```python
from build123d import *

# Parameters (mm, degrees)
F1_DEPTH = 17.5
F2_W     = 8
F2_H     = 3
F2_W_2   = 15
F2_H_2   = 1
F3_DEPTH = 50
F5_DEPTH = 2.5


# Not quite as in the source:
# - a pattern or mirror of a feature is missing from the dataset's text; its kind, count and spacing are read off the source's solid


with BuildPart() as f1:
    # F0 (on Front) → F1 (new body, symmetric)
    with BuildSketch(Plane.XZ):
        Polygon((-11.8, 0), (0, 0), (11.8, 0), (11.8, 8), (11, 8), (7.75, 2.5), (0, 2.5), (-7.75, 2.5), (-11, 8), (-11.8, 8), align=None)
    extrude(amount=F1_DEPTH, both=True)

    # F2 (on Right) → F3 (cut, symmetric)
    with BuildSketch(Plane.YZ):
        with Locations((0, 4)):
            Rectangle(F2_W, F2_H)
        with Locations((0, 0.5)):
            Rectangle(F2_W_2, F2_H_2)
    extrude(amount=F3_DEPTH, both=True, mode=Mode.SUBTRACT)

    # F4 (on Top) → F5 (join)
    with BuildSketch(Plane.XY):
        Polygon((26.4065545634, 26.1439538722), (11.8, 17.5), (11.8, 8.5), (27.6797758895, 23.9924642824), align=None)
        Polygon((11.8, -8.5), (11.8, -17.5), (21.2564246661, -23.0961793217), (23.2712739184, -19.6914867497), align=None)
    f5 = extrude(amount=F5_DEPTH)

    # F5_copies: F5 across plane
    add(f5.mirror(Plane(origin=(0, 0, 0), x_dir=(0, 0, -1), z_dir=(-1, 0, 0))))


solid = f1.part
```
Geometry: final body of the model. Coordinates: model frame, mm. A direction names the side the tool comes from. Round coordinates to 2 decimals unless told otherwise and drop trailing zeros. Order: outer loops, then holes, each group sorted by start corner. A loop starts at its lowest first (then second) coordinate and runs counter-clockwise, first axis right, second up. Notation, with made-up numbers: (62, 11) - (121, 11) arc R14 cw to (121, 22) - close; hole circle Ø6 at (57, 42). An arc over 180 degrees is marked (long way). Write item = value, one per line. Start each with the question number.
Q1. Cut plane B-B on z = 6.25. Return the cut outline in (x, y), and give its area (3 significant figures).
Q2. Ray query, line 1 (Z direction, x = -11, y = -2); line 2 (Z direction, x = 1, y = -8); line 3 (X direction, y = -6.5, z = 7.75). Return the intervals inside material, ascending. Write a range as from..to.
Q3. Cut plane D-D on y = -15.5. Return the cut outline in (x, z) (3 decimals).
Q4. Cut plane C-C on x = 17.5. Return the cut outline in (y, z), and give its area (3 significant figures).
Q5. Access query for faces 1 (the flat face through (19, 18, 2.5)), 2 (the flat face through (-16, -17, 2.5)), 3 (the flat face through (0, 0, 1)), 4 (the flat face through (-19.63, 16.14, 1.23)), 5 (the flat face through (17.616, -14.174, 1.232)). Directions: +Z, -Z, +X, -X, +Y, -Y. A direction counts if a zero-diameter tool reaches every point of the face in a straight line with its end or side. Return the directions, or none.
Q6. Cut plane A-A on y = 2. Return the cut outline in (x, z), and give its area (3 significant figures).
Q7. Pin query (flat end, axial travel): pin 1 (3.5 mm diameter, centred on x = 9.5, z = 4.5, fed in from +Y); pin 2 (5.5 mm diameter, centred on x = -17, y = -18.5, fed in from +Z); pin 3 (0.7 mm diameter, centred on x = 10.5, y = 1, fed in from -Z). Return the tip coordinate at first contact, or that it passes through.
Q8. Pull-direction query (Z, two-part tool) for faces 6 (the flat face through (11, 0, 5.5)), 7 (the flat face through (-16.46, -20.26, 1.23)), 8 (the flat face through (16, -17, 2.5)); classes: +Z half, -Z half, draft (parallel to the pull), parting line (faces both ways), or undercut.
Outcome:
q1.outline = (-11.8, -17.5) - (-9.97, -17.5) - (-9.97, 17.5) - (-11.8, 17.5) - close; (9.97, -17.5) - (11.8, -17.5) - (11.8, 17.5) - (9.97, 17.5) - close
q1.area = 128 mm^2
q2.line_1 = 1..2.5, 5.5..8
q2.line_2 = 0..2.5
q2.line_3 = -11.8..-10.85, 10.85..11.8
q3.outline = (-18.975, 0) - (18.975, 0) - (18.975, 2.5) - (11.8, 2.5) - (11.8, 8) - (11, 8) - (7.75, 2.5) - (-7.75, 2.5) - (-11, 8) - (-11.8, 8) - (-11.8, 2.5) - (-18.975, 2.5) - close
q4.outline = (-20.87, 0) - (-14.06, 0) - (-14.06, 2.5) - (-20.87, 2.5) - close; (14.06, 0) - (20.87, 0) - (20.87, 2.5) - (14.06, 2.5) - close
q4.area = 34.1 mm^2
q5.face_1 = +Z, +X, +Y, -Y
q5.face_2 = +Z, -X, +Y, -Y
q5.face_3 = -Z, +X, -X
q5.face_4 = +Z, -Z, -X
q5.face_5 = +Z, -Z, +X
q6.outline = (-11.8, 1) - (11.8, 1) - (11.8, 2.5) - (-11.8, 2.5) - close; (-11.8, 5.5) - (-9.52, 5.5) - (-11, 8) - (-11.8, 8) - close; (9.52, 5.5) - (11.8, 5.5) - (11.8, 8) - (11, 8) - close
q6.area = 43.1 mm^2
q7.pin_1 = 17.5
q7.pin_2 = 2.5
q7.pin_3 = 1
q8.face_6 = undercut
q8.face_7 = draft
q8.face_8 = +Z half
